Autodesk Inventor part; units mm, degrees
ref_plane "YZ Plane" through (0, 0, 0) normal (1, 0, 0) x (0, 1, 0)
ref_plane "XZ Plane" through (0, 0, 0) normal (0, 1, 0) x (-1, 0, 0)
ref_plane "XY Plane" through (0, 0, 0) normal (0, 0, 1) x (1, 0, 0)
sketch "Skizze1" plane through (0, 0, 0) normal (0, 0, 1) x (1, 0, 0)
  line L0 (15, 7.5) -> (15, -7.5)
  line L1 (15, -7.5) -> (-15, -7.5)
  line L2 (-15, -7.5) -> (-15, 7.5)
  line L3 (-15, 7.5) -> (15, -7.5) construction
  line L4 (15, 7.5) -> (-15, -7.5) construction
  arc A0 (-13, 7.5) -> (13, 7.5) centre (0, 7.5) ccw
  line L5 (-15, 7.5) -> (-13, 7.5)
  line L6 (13, 7.5) -> (15, 7.5)
  point P0 (0, 0)
  dimension "d0" = 30
  dimension "d1" = 15
  dimension "d2" = 26
extrude "Extrusion1" add sketch "Skizze1" along normal blind 132
sketch "Skizze2" plane through (-15, -7.5, 0) normal (-1, 0, 0) x (0, 0, 1)
  line L0 (0, 15) -> (0, 2)
  line L1 (58.5, 15) -> (66, 15)
  line L2 (0, 15) -> (132, 15)
  line L3 (73.5, 15) -> (73.5, 13)
  line L4 (73.5, 13) -> (58.5, 13)
  line L5 (58.5, 13) -> (58.5, 15)
  line L6 (58.5, 17) -> (73.5, 13) construction
  line L7 (73.5, 17) -> (58.5, 13) construction
  line L8 (58.5, 15) -> (73.5, 15)
  point P0 (0, 7.5)
  dimension "d5" = 66
extrude "Extrusion2" add sketch "Skizze2" along normal blind 15
sketch "Skizze3" plane through (15, -7.5, 0) normal (1, 0, 0) x (0, 0, -1)
  line L0 (-73.5, 15) -> (-73.5, 13)
  line L1 (-73.5, 13) -> (-58.5, 13)
  line L2 (-58.5, 13) -> (-58.5, 15)
  line L3 (-58.5, 17) -> (-73.5, 13) construction
  line L4 (-73.5, 17) -> (-58.5, 13) construction
  line L5 (-73.5, 15) -> (-58.5, 15)
  point P0 (0, 7.5)
  dimension "d11" = 15
  dimension "d12" = 4
extrude "Extrusion3" add sketch "Skizze3" along normal blind 15
sketch "Skizze4" plane through (13, 7.5, 132) normal (0, 1, 0) x (1, 0, 0)
  line L0 (2, 58.5) -> (17, 58.5)
  line L1 (2, 73.5) -> (2, 58.5)
  line L2 (2, 73.5) -> (17, 73.5)
  circle A0 centre (9.5, 66) radius 2.5
  line L3 (-28, 58.5) -> (-28, 73.5)
  line L4 (-28, 73.5) -> (-43, 73.5)
  circle A1 centre (-35.5, 66) radius 2.5
  point P0 (-13, 132)
  point P1 (-43, 58.5)
  dimension "d15" = 5
  dimension "d16" = 5
extrude "Extrusion4" cut sketch "Skizze4" against normal blind 15
sketch "Skizze5" plane through (0, 0, 0) normal (0, 0, -1) x (-1, 0, 0)
  line L0 (15, -7.5) -> (-15, -7.5)
  line L1 (-15, -7.5) -> (15, -7.5)
  line L2 (15, -7.5) -> (15, 22.5)
  line L3 (15, 22.5) -> (-15, 22.5)
  line L4 (-15, 22.5) -> (-15, -7.5)
  point P0 (0, 0)
  dimension "d19" = 30
  dimension "d20" = 30
extrude "Extrusion5" add sketch "Skizze5" along normal blind 2
sketch "Skizze6" plane through (0, 0, 132) normal (0, 0, 1) x (1, 0, 0)
  line L0 (-15, -7.5) -> (15, -7.5)
  line L1 (15, -7.5) -> (15, 22.5)
  line L2 (15, 22.5) -> (-15, 22.5)
  line L3 (-15, 22.5) -> (-15, -7.5)
  point P0 (0, 0)
  dimension "d23" = 30
  dimension "d24" = 30
extrude "Extrusion6" add sketch "Skizze6" along normal blind 2
sketch "Skizze7" plane through (0, 0, 134) normal (0, 0, 1) x (1, 0, 0)
  arc A0 (-13, 7.5) -> (13, 7.5) centre (0, 7.5) ccw
  circle A1 centre (0, 7.5) radius 3.75
  point P0 (0, 0)
  dimension "d27" = 7.5
extrude "Extrusion7" cut sketch "Skizze7" against normal through all
fillet "Rundung1" radius 3 1 edges at (15, 22.5, 133)
fillet "Rundung2" radius 3 1 edges at (-15, 22.5, 133)
fillet "Rundung3" radius 3 1 edges at (-15, 22.5, -1)
fillet "Rundung4" radius 3 1 edges at (15, 22.5, -1)
properties part number "Motorhalterung_Teil1.1"
Design review of the part built by this model. Coordinates are the model's own, in mm. A direction names the side the tool comes from. Coordinates: 2 decimals unless noted, no trailing zeros. Loops run counter-clockwise (first coordinate to the right, second up) from the corner with the lowest first, then second, coordinate; pieces in that order, holes last. Notation, with made-up numbers: (19.5, 31) -> (52.5, 31) arc R7 ccw to (52.5, 39) -> close; hole circle Ø11 at (80, 12.25). An arc over 180 degrees is marked (long way). Answer as a JSON object with one key per item and string values.
Q1. Take a section at A-A on x = 22.5. Give the boundary of the cut face in (y, z), plus the area to 3 significant figures.
Answer block:
{"outline": "(5.5, 58.5) -> (7.5, 58.5) -> (7.5, 63.5) -> (5.5, 63.5) -> close; (5.5, 68.5) -> (7.5, 68.5) -> (7.5, 73.5) -> (5.5, 73.5) -> close", "area": "20.0 mm^2"}
Q2. Take a section at B-B on z = 66. Give the boundary of the cut face in (x, y), plus the area to 3 significant figures.
Answer block:
{"outline": "(-30, 5.5) -> (-25, 5.5) -> (-25, 7.5) -> (-30, 7.5) -> close; (-20, 5.5) -> (-15, 5.5) -> (-15, -7.5) -> (15, -7.5) -> (15, 5.5) -> (20, 5.5) -> (20, 7.5) -> (13, 7.5) arc R13 cw to (-13, 7.5) -> (-20, 7.5) -> close; (25, 5.5) -> (30, 5.5) -> (30, 7.5) -> (25, 7.5) -> close", "area": "225 mm^2"}
Q3. Take a section at D-D on x = 0. Give the boundary of the cut face in (y, z), plus the area to 3 significant figures.
Answer block:
{"outline": "(-7.5, -2) -> (3.75, -2) -> (3.75, 0) -> (-5.5, 0) -> (-5.5, 132) -> (3.75, 132) -> (3.75, 134) -> (-7.5, 134) -> close; (11.25, -2) -> (22.5, -2) -> (22.5, 0) -> (11.25, 0) -> close; (11.25, 132) -> (22.5, 132) -> (22.5, 134) -> (11.25, 134) -> close", "area": "354 mm^2"}
Q4. Clearance check with flat-ended pins moving along their axes: pin 1 Ø6 at (y, z) = (-0.5, 77.5) entering from -X; pin 2 Ø0.6 at (x, y) = (24.5, 6.5) entering from +Z; pin 3 Ø10 at (x, z) = (-4, 95) entering from +Y. State where each tip first meets the part, or that it passes through.
Answer block:
{"pin 1": "stops at x = -15", "pin 2": "stops at z = 73.5", "pin 3": "stops at y = -1.88"}
Q5. To check wall thickness, follow L1, parallel to X at y = 6.9, z = 66; L2, parallel to Z at x = 22.5, y = 6; L3, parallel to Z at x = 8.5, y = 14.5. State the ranges of each line that lie inside material, in increasing order.
Answer block:
{"L1": "x = -30 to -25, -20 to -12.99, 12.99 to 20, 25 to 30", "L2": "z = 58.5 to 63.5, 68.5 to 73.5", "L3": "z = -2 to 0, 132 to 134"}
Q6. Take a section at C-C on y = 14. Give the boundary of the cut face in (x, z), plus the area to 3 significant figures.
Answer block:
{"outline": "(-15, -2) -> (15, -2) -> (15, 0) -> (-15, 0) -> close; (-15, 132) -> (15, 132) -> (15, 134) -> (-15, 134) -> close", "area": "120 mm^2"}
Q7. The part is to be moulded in two halves that separate along X. For faces 5 (the flat face through (0, 12, 132)), 6 (the flat face through (18, 7.5, 66)), 7 (the cylindrical face through (-14.1, 21.64, 133.01)), say which applies: +X half, -X half, draft (parallel to the pull), parting line (faces both ways), or undercut.
Answer block:
{"face 5": "undercut", "face 6": "draft", "face 7": "-X half"}
Q8. Tool access review of faces 1 (the flat face through (19, 5.5, 66)), 2 (the cylindrical face through (0.286, -5.497, 65.076)), 3 (the flat face through (-18, 7.5, 66)), 4 (the flat face through (-19, 5.5, 66)): name each direction out of +Z, -Z, +X, -X, +Y, -Y from which nothing blocks a thin tool from reaching the whole face with its end or side.
Answer block:
{"face 1": "+Z, -Z, +X, -Y", "face 2": "+Y", "face 3": "+X, -X, +Y", "face 4": "+Z, -Z, -X, -Y"}
